Here's how the part is built. I have some questions about the finished solid (model axes, mm). Face numbers are marked on the shaded views. Round coordinates to 2 decimals unless told otherwise and drop trailing zeros. Order: outer loops, then holes, each group sorted by start corner. A loop starts at its lowest first (then second) coordinate and runs counter-clockwise, first axis right, second up.
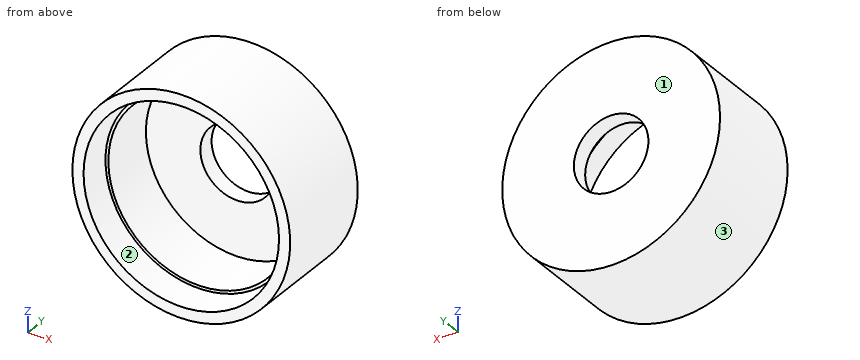
Autodesk Inventor part; units mm, degrees
ref_plane "YZ Plane" through (0, 0, 0) normal (1, 0, 0) x (0, 1, 0)
ref_plane "XZ Plane" through (0, 0, 0) normal (0, 1, 0) x (-1, 0, 0)
ref_plane "XY Plane" through (0, 0, 0) normal (0, 0, 1) x (1, 0, 0)
sketch "Boceto4" plane through (0, 0, 0) normal (0, 1, 0) x (-1, 0, 0)
  circle A0 centre (0, 0) radius 17.05
  circle A1 centre (0, 0) radius 19
  dimension "d10" = 34.1
  dimension "d11" = 38
extrude "Extrusión4" add sketch "Boceto4" against normal blind 18
sketch "Boceto5" plane through (0, 0, 0) normal (0, 1, 0) x (1, 0, 0)
  circle A0 centre (0, 0) radius 17.05
extrude "Extrusión5" add sketch "Boceto5" against normal blind 3
sketch "Boceto6" plane through (0, -3, 0) normal (0, -1, 0) x (1, 0, 0)
  circle A0 centre (0, 0) radius 6.5
  dimension "d16" = 13
extrude "Extrusión6" cut sketch "Boceto6" against normal blind 3
sketch "Boceto7" plane through (0, -3, 0) normal (0, -1, 0) x (1, 0, 0)
  circle A0 centre (0, 0) radius 16
  circle A1 centre (0, 0) radius 6.5
  circle A2 centre (0, 0) radius 16.5
  dimension "d19" = 32
  dimension "d20" = 33
extrude "Extrusión7" add sketch "Boceto7" along normal blind 10 contours A2
properties part number "tapa seccion alimentacion"
1. If we section it at A-A, the plane x = 0: Write out the boundary of the cut face in (y, z).
Evaluation:
outline: (-18, -19) - (0, -19) - (0, -6.5) - (-3, -6.5) - (-3, -16) - (-13, -16) - (-13, -16.5) - (-3, -16.5) - (-3, -17.05) - (-18, -17.05) - close; (-18, 17.05) - (-3, 17.05) - (-3, 16.5) - (-13, 16.5) - (-13, 16) - (-3, 16) - (-3, 6.5) - (0, 6.5) - (0, 19) - (-18, 19) - close
2. If we section it at B-B, the plane z = 0: Write out the boundary of the cut face in (x, y).
Evaluation:
outline: (-19, -18) - (-17.05, -18) - (-17.05, -3) - (-16.5, -3) - (-16.5, -13) - (-16, -13) - (-16, -3) - (-6.5, -3) - (-6.5, 0) - (-19, 0) - close; (6.5, -3) - (16, -3) - (16, -13) - (16.5, -13) - (16.5, -3) - (17.05, -3) - (17.05, -18) - (19, -18) - (19, 0) - (6.5, 0) - close
3. I'm going to push flat-ended pins straight in: P1, Ø4, axis at y = -5.5, z = 13.5, coming from the -X side; P2, Ø6, axis at x = -4, y = -11, coming from the +Z side; P3, Ø17, axis at x = -7, z = -1, coming from the -Y side. Where does each tip first touch, or does it pass through?
Evaluation:
P1: stops at x = -15.12
P2: stops at z = 18.97
P3: stops at y = -3
4. I need wall thicknesses on probe 1 along Z at (x, y) = (0, -8.25); probe 2 along Z at (x, y) = (0, -1.05); probe 3 along Z at (x, y) = (0, -14.75). Which ranges of each line are inside material? Lowest first, please.
Evaluation:
probe 1: z = -19 to -17.05, -16.5 to -16, 16 to 16.5, 17.05 to 19
probe 2: z = -19 to -6.5, 6.5 to 19
probe 3: z = -19 to -17.05, 17.05 to 19
5. If we section it at D-D, the plane z = -9.5: Write out the boundary of the cut face in (x, y).
Evaluation:
outline: (-16.45, -18) - (-14.16, -18) - (-14.16, -3) - (-13.49, -3) - (-13.49, -13) - (-12.87, -13) - (-12.87, -3) - (12.87, -3) - (12.87, -13) - (13.49, -13) - (13.49, -3) - (14.16, -3) - (14.16, -18) - (16.45, -18) - (16.45, 0) - (-16.45, 0) - close
6. If we mould it in two halves opening along X, with no side actions, what happens to the marked faces 1, 2 and 3? For each: released by +X, released by -X, zero draft, split by the parting line, or undercut.
Evaluation:
face 1: zero draft
face 2: undercut
face 3: split by the parting line
7. If we section it at C-C, the plane y = -10.5: Write out the boundary of the cut face in (x, z), and give its area (3 significant figures).
Evaluation:
outline: circle Ø38 at (0, 0); circle Ø33 at (0, 0); hole circle Ø34.1 at (0, 0); hole circle Ø32 at (0, 0)
area: 272 mm2
